For this review, take the finished solid that the model builds, in its own axes (mm). A direction names the side the tool comes from. Round coordinates to 2 decimals unless told otherwise and drop trailing zeros. Order: outer loops, then holes, each group sorted by start corner. A loop starts at its lowest first (then second) coordinate and runs counter-clockwise, first axis right, second up. Notation, with made-up numbers: (66, 12) -> (106, 12) arc R11 cw to (106, 27) -> close; hole circle Ø6 at (12.25, -15.5). An arc over 180 degrees is marked (long way). Use a Markdown table: item, result. Add a question column.
1) Consider section A-A (y = 183.5). State the section outline as (x, z) points.
2) Consider section C-C (x = -83.5). State the section outline as (y, z) points, plus the area to 3 significant figures.
3) Wall thickness on line 1 along Y through (x, z) = (151, 168); line 2 along X through (y, z) = (141, -179); line 3 along Z through (x, y) = (147.5, 109.5): over which ranges is each line inside the solid? List them lowest first. Write a range as [from, to].
4) Draft analysis for pull direction Z (two halves, no side actions). For faces 5 (the face through (-194.8, 101.5, 112.3)), 6 (the face through (194.8, 101.5, -112.3)), 7 (the face through (187, 2.54, 81)), state which applies: pulls with the +Z half, pulls with the -Z half, needs draft (parallel to the pull), parting line crosses it, or undercut.
5) Consider section D-D (x = -238.5). State the section outline as (y, z) points.
6) Machinability: for faces 1 (the face through (212, 2.54, -93)), 2 (the face through (170.859, 1.252, 100.496)), 3 (the face through (194.668, 101.465, 112.528)), 4 (the face through (-194.668, 101.465, -112.528)), which of the approach directions +Z, -Z, +X, -X, +Y, -Y give a long, thin tool a straight path to every point of the face, cutting with its end or side? Answer none if there is none.
7) Consider section B-B (z = -61.5). State the section outline as (x, y) points.
8) Clearance check with flat-ended pins moving along their axes: P1, Ø1.5, axis at x = -155, y = 148.5, coming from the -Z side; P2, Ø6, axis at y = 174.5, z = -150, coming from the +X side; P3, Ø3, axis at x = 192, y = 64, coming from the -Z side. State where each tip first meets the part, or that it passes through.
```python
from build123d import *

# Parameters (mm, degrees)
BOSS_EXTRUDE1_DEPTH = 2.54
BOSS_EXTRUDE2_DEPTH = 203.2


with BuildPart() as part:
    # Sketch1 → Boss-Extrude1 (new body)
    with BuildSketch(Plane(origin=(0, 0, 0), x_dir=(1, 0, 0), z_dir=(0, 1, 0))):
        Polygon((143.769509274, -249.016094641), (287.539018547, 0), (143.769509274, 249.016094641), (-143.769509274, 249.016094641), (-287.539018547, 0), (-143.769509274, -249.016094641), align=None)
        Polygon((114.440115599, -198.216094641), (228.880231198, 0), (114.440115599, 198.216094641), (-114.440115599, 198.216094641), (-228.880231198, 0), (-114.440115599, -198.216094641), align=None, mode=Mode.SUBTRACT)
    extrude(amount=BOSS_EXTRUDE1_DEPTH)

    # Sketch2 → Boss-Extrude2 (add)
    with BuildSketch(Plane(origin=(0, 0, 0), x_dir=(1, 0, 0), z_dir=(0, 1, 0))):
        Polygon((128.11073119, 225.819195391), (-131.509794276, 223.856745403), (-259.620525466, -1.962449988), (-128.11073119, -225.819195391), (131.509794276, -223.856745403), (259.620525466, 1.962449988), align=None)
        Polygon((125.21627381, 220.717171301), (-128.538540494, 218.799059737), (-253.754814303, -1.918111564), (-125.21627381, -220.717171301), (128.538540494, -218.799059737), (253.754814303, 1.918111564), align=None, mode=Mode.SUBTRACT)
    extrude(amount=BOSS_EXTRUDE2_DEPTH)


solid = part.part
```
Results list:
| question | item | result |
|---|---|---|
| 1 | outline | (-259.62, 1.96) -> (-131.51, -223.86) -> (128.11, -225.82) -> (259.62, -1.96) -> (131.51, 223.86) -> (-128.11, 225.82) -> close; hole (-253.75, 1.92) -> (-128.54, -218.8) -> (125.22, -220.72) -> (253.75, -1.92) -> (128.54, 218.8) -> (-125.22, 220.72) -> close |
| 2 | outline | (0, -249.02) -> (2.54, -249.02) -> (2.54, -224.22) -> (203.2, -224.22) -> (203.2, -219.14) -> (2.54, -219.14) -> (2.54, -198.22) -> (0, -198.22) -> close; (0, 198.22) -> (2.54, 198.22) -> (2.54, 220.4) -> (203.2, 220.4) -> (203.2, 225.48) -> (2.54, 225.48) -> (2.54, 249.02) -> (0, 249.02) -> close |
| 2 | area | 2,300 mm2 |
| 3 | line 1 | [0, 2.54] |
| 3 | line 2 | [-156.96, -151.12], [149.72, 155.62] |
| 3 | line 3 | [-192.81, -182.79], [185.38, 195.67] |
| 4 | face 5 | pulls with the +Z half |
| 4 | face 6 | pulls with the -Z half |
| 4 | face 7 | undercut |
| 5 | outline | (0, -84.94) -> (2.54, -84.94) -> (2.54, -35.27) -> (203.2, -35.27) -> (203.2, -24.97) -> (2.54, -24.97) -> (2.54, 27.88) -> (203.2, 27.88) -> (203.2, 37.91) -> (2.54, 37.91) -> (2.54, 84.94) -> (0, 84.94) -> close |
| 6 | face 1 | +Y |
| 6 | face 2 | +Y, -Y |
| 6 | face 3 | +Z, +X, +Y |
| 6 | face 4 | -Z, -X, +Y |
| 7 | outline | (-252.03, 0) -> (-193.37, 0) -> (-193.37, 2.54) -> (-217.78, 2.54) -> (-217.78, 203.2) -> (-223.62, 203.2) -> (-223.62, 2.54) -> (-252.03, 2.54) -> close; (193.37, 0) -> (252.03, 0) -> (252.03, 2.54) -> (224.64, 2.54) -> (224.64, 203.2) -> (218.75, 203.2) -> (218.75, 2.54) -> (193.37, 2.54) -> close |
| 8 | P1 | z = -183.77 |
| 8 | P2 | x = 174.41 |
| 8 | P3 | z = -119.62 |
